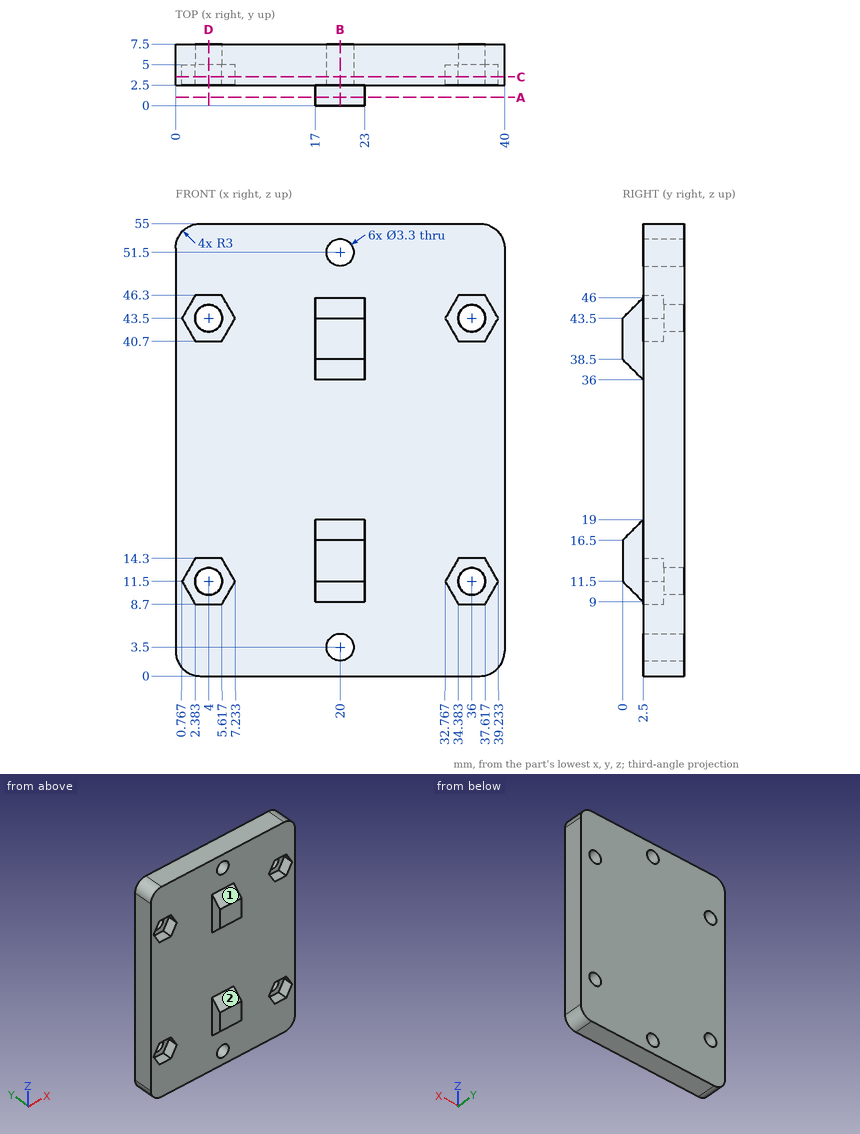
Here's the drawing with two shaded views (mm, measured from the low corner). I have some questions. A direction names the side the tool comes from. Give positions to 0.01 mm unless a question says otherwise; leave off trailing zeros. Write each loop counter-clockwise with the first axis right and the second up, starting at its lowest first coordinate (ties: lowest second). Pieces come first, ordered by that corner, then holes. Notation, with made-up numbers: (23.5, -14.5) -> (54.5, -14.5) arc R25 ccw to (54.5, 10.5) -> close; hole circle Ø9 at (88.25, 61). An arc over 180 degrees is marked (long way). Use one line per item in the form item = value.
1) Suppose I cut it at C-C (y = 3.5). Give the number of separate pieces and of enclosed holes in the cut face, and give its area (3 significant figures).
Verdict:
separate_pieces = 1
enclosed_holes = 6
area = 2,070 mm2
2) Suppose I cut it at D-D (x = 4). Please give me the cut outline in (y, z).
Verdict:
outline = (2.5, 0) -> (7.5, 0) -> (7.5, 9.85) -> (5, 9.85) -> (5, 8.7) -> (2.5, 8.7) -> close; (2.5, 14.3) -> (5, 14.3) -> (5, 13.15) -> (7.5, 13.15) -> (7.5, 41.85) -> (5, 41.85) -> (5, 40.7) -> (2.5, 40.7) -> close; (2.5, 46.3) -> (5, 46.3) -> (5, 45.15) -> (7.5, 45.15) -> (7.5, 55) -> (2.5, 55) -> close
3) Suppose I cut it at B-B (x = 20). Please give me the cut outline in (y, z).
Verdict:
outline = (0, 11.5) -> (2.5, 9) -> (2.5, 5.15) -> (7.5, 5.15) -> (7.5, 49.85) -> (2.5, 49.85) -> (2.5, 46) -> (0, 43.5) -> (0, 38.5) -> (2.5, 36) -> (2.5, 19) -> (0, 16.5) -> close; (2.5, 0) -> (7.5, 0) -> (7.5, 1.85) -> (2.5, 1.85) -> close; (2.5, 53.15) -> (7.5, 53.15) -> (7.5, 55) -> (2.5, 55) -> close
4) Suppose I cut it at A-A (y = 1). Please give me the cut outline in (x, z).
Verdict:
outline = (17, 10.5) -> (23, 10.5) -> (23, 17.5) -> (17, 17.5) -> close; (17, 37.5) -> (23, 37.5) -> (23, 44.5) -> (17, 44.5) -> close
5) On a 3-axis mill with a long thin cutter (end or side, diameter ignored), from which of +Z, -Z, +X, -X, +Y, -Y can I reach the whole of each face in a straight line? I mean the marked faces 1 and 2. Say none if no direction works.
Verdict:
face_1 = +Z, +X, -X, -Y
face_2 = +X, -X, -Y
6) I'm going to push flat-ended pins straight in: pin 1 (0.7 mm diameter, centred on x = 36, y = 3.5, fed in from -Z); pin 2 (4 mm diameter, centred on x = 20, z = 51.5, fed in from -Y); pin 3 (1.3 mm diameter, centred on y = 1.5, z = 12.5, fed in from +X); pin 4 (5.5 mm diameter, centred on x = 36, z = 11.5, fed in from -Y). Where does each tip first touch, or does it pass through?
Verdict:
pin_1 = 0
pin_2 = 2.5
pin_3 = 23
pin_4 = 5
7) If I drill on L1, parallel to X at y = 6.75, z = 43.5; L2, parallel to Z at x = 4, y = 6.25; L3, parallel to Z at x = 20, y = 4.4, over which ranges is the centre line in solid material (lowest first)? Write a range as [from, to].
Verdict:
L1 = [0, 2.35], [5.65, 34.35], [37.65, 40]
L2 = [0, 9.85], [13.15, 41.85], [45.15, 55]
L3 = [0, 1.85], [5.15, 49.85], [53.15, 55]
